Read the model definition and answer for the solid it produces. Units are mm, in the model's axes. A direction names the side the tool comes from. Coordinates: 2 decimals unless noted, no trailing zeros. Order: outer loops, then holes, each group sorted by start corner. A loop starts at its lowest first (then second) coordinate and runs counter-clockwise, first axis right, second up. Notation, with made-up numbers: M 7.5,83 L 52.5,83 A22 ccw 52.5,101 Z; hole C -37.5,11 d2. An arc over 180 degrees is marked long. Put each result on its own line as item: value.
from build123d import *

# Parameters (mm, degrees)
SKETCH1_R           = 1.3
SKETCH1_R_2         = 0.3
BOSS_EXTRUDE1_DEPTH = 1
SKETCH1_3_R         = 0.765
BOSS_EXTRUDE2_DEPTH = 0.7
BOSS_EXTRUDE3_DEPTH = 0.6
BOSS_EXTRUDE4_DEPTH = 0.6
BOSS_EXTRUDE5_DEPTH = 0.4
SKETCH6_R           = 0.3
BOSS_EXTRUDE6_DEPTH = 0.4


with BuildPart() as part:
    # Sketch1 → Boss-Extrude1 (new body, symmetric)
    with BuildSketch(Plane.XY):
        Circle(SKETCH1_R)
        Circle(SKETCH1_R_2, mode=Mode.SUBTRACT)
    extrude(amount=BOSS_EXTRUDE1_DEPTH, both=True)



with BuildPart() as body_2:
    # Sketch1_3 → Boss-Extrude2 (new body, symmetric)
    with BuildSketch(Plane.XY):
        with Locations((3.98, -0.682)):
            Circle(SKETCH1_3_R)
    extrude(amount=BOSS_EXTRUDE2_DEPTH, both=True)


with BuildPart() as part_1:
    add(part.part)

    add(body_2.part)  # Boss-Extrude3 merges body 2
    # Sketch1_4 → Boss-Extrude3 (add, symmetric)
    with BuildSketch(Plane.XY):
        with BuildLine():
            ThreePointArc((3.590115999, -1.340191056), (3.217046127, -0.626085884), (3.690239158, 0.025999756))
            Line((3.690239158, 0.025999756), (1.766699303, 0.999180984))
            Line((1.766699303, 0.999180984), (0.233288639, 1.27889656))
            ThreePointArc((0.233288639, 1.27889656), (0.998317392, 0.832683844), (1.3, 0))
            ThreePointArc((1.3, 0), (1.084853213, -0.716305456), (0.510625375, -1.195517347))
            ThreePointArc((0.510625375, -1.195517347), (2.066949931, -0.914952316), (3.590115999, -1.340191056))
        make_face()
    extrude(amount=BOSS_EXTRUDE3_DEPTH, both=True)

    # Sketch1_5 → Boss-Extrude4 (add, symmetric)
    with BuildSketch(Plane.XY):
        with BuildLine():
            ThreePointArc((-1.295848634, -0.103809043), (-1.071749439, 0.735767042), (-0.368782161, 1.24659525))
            Line((-0.368782161, 1.24659525), (-1.279338258, 1.931105297))
            Line((-1.279338258, 1.931105297), (-3.469420101, 2.791170079))
            Line((-3.469420101, 2.791170079), (-3.851452989, 2.234684794))
            Line((-3.851452989, 2.234684794), (-2.261840722, 0.499950592))
            Line((-2.261840722, 0.499950592), (-1.295848634, -0.103809043))
        make_face()
    extrude(amount=BOSS_EXTRUDE4_DEPTH, both=True)



with BuildPart() as body_2_2:
    # Sketch2 → Revolve1 (revolve)
    with BuildSketch(Plane.XY):
        with BuildLine():
            Line((-3.851452989, 2.234684794), (-3.443951242, 2.828269098))
            Line((-3.443951242, 2.828269098), (-3.769598187, 3.051829084))
            Line((-3.769598187, 3.051829084), (-4.833144721, 1.502622153))
            ThreePointArc((-4.833144721, 1.502622153), (-4.430488377, 1.507175235), (-4.298614364, 1.887651393))
            Line((-4.298614364, 1.887651393), (-3.851452989, 2.234684794))
        make_face()
    revolve(axis=Axis((-3.769598187, 3.051829084, 0), (-0.565974648, -0.824422645, 0)))


with BuildPart() as part_2:
    add(part_1.part)

    add(body_2_2.part)  # Revolve2 merges body 2 2
    # Sketch4 → Revolve2 (revolve)
    with BuildSketch(Plane.XY):
        Polygon((-3.68969938, 3.174750981), (-4.303268205, 2.281000641), (-5.053492813, 2.796037571), (-4.439923988, 3.68978791), align=None)
    revolve(axis=Axis((-3.68969938, 3.174750981, 0), (-0.565974648, -0.824422645, 0)))

    # Sketch5 → Boss-Extrude5 (add)
    with BuildSketch(Plane(origin=(0.299434714, 0.436169287, 0), x_dir=(0.824422645, -0.565974648, 0), z_dir=(0.565974648, 0.824422645, 0))):
        Polygon((-4.838700292, 0.75055535), (-5.488700292, 0.375277675), (-5.488700292, -0.375277675), (-4.838700292, -0.75055535), (-4.188700292, -0.375277675), (-4.188700292, 0.375277675), align=None)
    extrude(amount=BOSS_EXTRUDE5_DEPTH)

    # Sketch6 → Boss-Extrude6 (add)
    with BuildSketch(Plane(origin=(0.525824573, 0.765938345, 0), x_dir=(0.824422645, -0.565974648, 0), z_dir=(0.565974648, 0.824422645, 0))):
        with Locations((-4.838700292, 0)):
            Circle(SKETCH6_R)
    extrude(amount=BOSS_EXTRUDE6_DEPTH)


solid = part_2.part
Q1. Consider line 1 along Y through (x, z) = (0, -0.2); line 2 along Z through (x, y) = (-1.75, 1.6); line 3 along X through (y, z) = (-1.1, 0.95). Determine where each line is inside the solid, lowest interval first.
Answers below:
line 1: y = -1.3 to -0.3, 0.3 to 1.3
line 2: z = -0.6 to 0.6
line 3: x = -0.69 to 0.69
Q2. Given pin 1 (0.8 mm diameter, centred on x = 2, y = 0.5, fed in from +Z); pin 2 (0.5 mm diameter, centred on x = 4, y = -1, fed in from -Z); pin 3 (1.2 mm diameter, centred on x = 4, y = -0.5, fed in from +Z), each flat-ended and moving along its own axis, determine where each tip first touches the part or whether it passes through.
Answers below:
pin 1: stops at z = 0.6
pin 2: stops at z = -0.7
pin 3: stops at z = 0.7
Q3. Find section A-A on x = 0. Write down the section's boundary in (y, z), plus the area to 3 significant figures.
Answers below:
outline: M -1.3,-1 L -0.3,-1 L -0.3,1 L -1.3,1 Z; M 0.3,-1 L 1.3,-1 L 1.3,1 L 0.3,1 Z
area: 4.00 mm^2
Q4. A tool of negligible diameter and unlimited length cuts with its end or side. For faces 1 (the face through (-1.03, -0.79, 0.01)), 2 (the face through (4, -1, -0.7)), 3 (the face through (4, -1, 0.7)), from which of +Z, -Z, +X, -X, +Y, -Y can it reach the whole face along a straight path? Write none if from no direction.
Answers below:
face 1: none
face 2: -Z, +X, +Y, -Y
face 3: +Z, +X, +Y, -Y
Q5. Find section C-C on x = 3.98. Write down the section's boundary in (y, z), plus the area to 3 significant figures.
Answers below:
outline: M -1.45,-0.7 L 0.08,-0.7 L 0.08,0.7 L -1.45,0.7 Z
area: 2.14 mm^2
Q6. Find section D-D on x = 3. Write down the section's boundary in (y, z).
Answers below:
outline: M -1.09,-0.6 L 0.38,-0.6 L 0.38,0.6 L -1.09,0.6 Z
Q7. Find section B-B on y = -0.5. Write down the section's boundary in (x, z), plus the area to 3 significant figures.
Answers below:
outline: M -1.2,-1 L 1.2,-1 L 1.2,-0.6 L 3.24,-0.6 L 3.24,-0.7 L 4.72,-0.7 L 4.72,0.7 L 3.24,0.7 L 3.24,0.6 L 1.2,0.6 L 1.2,1 L -1.2,1 Z
area: 9.32 mm^2
